```python
from build123d import *

# Parameters (mm, degrees)
SKETCH1_W                                           = 15.5
SKETCH1_H                                           = 25
BOSS_EXTRUDE1_DEPTH                                 = 600
FILLET1_R                                           = 5
F_5_0MM_DOWEL_HOLE1_D                               = 6.6
F_5_0MM_DOWEL_HOLE1_DEPTH                           = 12
F_5_0MM_DOWEL_HOLE1_TIP                             = 1.982840043
CBORE_FOR_M5_HEX_SOCKET_HEAD_CAP_SCREW1_D           = 5.5
CBORE_FOR_M5_HEX_SOCKET_HEAD_CAP_SCREW1_CBORE_D     = 10
CBORE_FOR_M5_HEX_SOCKET_HEAD_CAP_SCREW1_CBORE_DEPTH = 5.4


with BuildPart() as part:
    # Sketch1 → Boss-Extrude1 (new body)
    with BuildSketch(Plane(origin=(0, 0, 0), x_dir=(1, 0, 0), z_dir=(0, 1, 0))):
        Rectangle(SKETCH1_W, SKETCH1_H)
    extrude(amount=BOSS_EXTRUDE1_DEPTH)

    # Fillet1
    fillet1_edges = [part.edges().sort_by_distance(p)[0] for p in [
        (0, 600, 12.5),
        (0, 600, -12.5),
    ]]
    fillet(fillet1_edges, radius=FILLET1_R)

    # Ø5.0mm Dowel Hole1
    with Locations(Plane(origin=(0, 0, 0), x_dir=(-1, 0, 0), z_dir=(0, -1, 0))):
        with Locations((0, 0)):
            Hole(F_5_0MM_DOWEL_HOLE1_D / 2, depth=F_5_0MM_DOWEL_HOLE1_DEPTH)
            with Locations((0, 0, -(F_5_0MM_DOWEL_HOLE1_DEPTH + F_5_0MM_DOWEL_HOLE1_TIP / 2))):  # 118° drill point
                Cone(0, F_5_0MM_DOWEL_HOLE1_D / 2, F_5_0MM_DOWEL_HOLE1_TIP, mode=Mode.SUBTRACT)

    # CBORE for M5 Hex Socket Head Cap Screw1 (through all)
    with Locations(Plane(origin=(7.75, 0, 0), x_dir=(0, 0, -1), z_dir=(1, 0, 0))):
        with Locations((0, 222), (0, 551), (0, 64)):
            CounterBoreHole(CBORE_FOR_M5_HEX_SOCKET_HEAD_CAP_SCREW1_D / 2, CBORE_FOR_M5_HEX_SOCKET_HEAD_CAP_SCREW1_CBORE_D / 2, CBORE_FOR_M5_HEX_SOCKET_HEAD_CAP_SCREW1_CBORE_DEPTH)


solid = part.part
```
Geometry check sheet. Reference: the model listing, model coordinates, mm. A direction names the side the tool comes from. Round coordinates to 2 decimals unless told otherwise and drop trailing zeros. Use a Markdown table: item, result.
Q1. Draft check along Y on faces 1 (the cylindrical face through (5.088, 555.957, 0.651)), 2 (the flat face through (2, 0, -3)), 3 (the flat face through (0, 293, 12.5)), 4 (the flat face through (0, 600, 0)). Enter one of: released by +Y, released by -Y, zero draft, split by the parting line, or undercut.
Solutions:
| item | result |
|---|---|
| face 1 | undercut |
| face 2 | released by -Y |
| face 3 | zero draft |
| face 4 | released by +Y |
Q2. Material ranges on line 1 (Y direction, x = -6.25, z = -0.5); line 2 (Y direction, x = 5.7, z = 0); line 3 (Z direction, x = 0, y = 7.25), recorded low to high.
Solutions:
| item | result |
|---|---|
| line 1 | y = 0 to 61.3, 66.7 to 219.3, 224.7 to 548.3, 553.7 to 600 |
| line 2 | y = 0 to 59, 69 to 217, 227 to 546, 556 to 600 |
| line 3 | z = -12.5 to -3.3, 3.3 to 12.5 |
Q3. Go/stop test with flat-tipped pins: P1, Ø5, axis at y = 549.5, z = -1.5, coming from the +X side; P2, Ø1.5, axis at x = 0.5, z = 10, coming from the +Y side; P3, Ø13, axis at y = 64, z = 0, coming from the -X side; P4, Ø3.5, axis at y = 551, z = 0, coming from the -X side (3 decimals). Record where each tip stops, or that it passes through.
Solutions:
| item | result |
|---|---|
| P1 | stops at x = 2.35 |
| P2 | stops at y = 599.68 |
| P3 | stops at x = -7.75 |
| P4 | passes through |
Q4. Access from +Z, -Z, +X, -X, +Y, -Y to the whole of each face (thin tool, end or side, straight path). Record for faces 5 (the flat face through (7.75, 296, 0)), 6 (the flat face through (2.35, 61.8, -2.2)).
Solutions:
| item | result |
|---|---|
| face 5 | +Z, -Z, +X, +Y, -Y |
| face 6 | +X |
